from build123d import *

# Parameters (mm, degrees)
SKETCH1_W            = 8.5
SKETCH1_H            = 8.5
BOSS_EXTRUDE1_DEPTH  = 5
SKETCH2_W            = 8.5
SKETCH2_H            = 8.5
BOSS_EXTRUDE2_DEPTH  = 2
SKETCH3_R            = 1.5
CUT_EXTRUDE1_DEPTH   = 2
SKETCH4_W            = 82
SKETCH4_H            = 8.5
BOSS_EXTRUDE3_DEPTH  = 3
SKETCH5_W            = 7
SKETCH5_H            = 8.5
BOSS_EXTRUDE4_DEPTH  = 8.5
CUT_EXTRUDE2_DEPTH   = 5
SKETCH7_R            = 1.5
CUT_EXTRUDE3_DEPTH   = 5
CUT_EXTRUDE4_DEPTH   = 10
SKETCH9_W            = 8.5
SKETCH9_H            = 8.5
SKETCH9_R            = 1.5
BOSS_EXTRUDE5_DEPTH  = 2
CUT_EXTRUDE5_DEPTH   = 2
SKETCH11_W           = 8.5
SKETCH11_H           = 8.5
SKETCH11_R           = 1.5
BOSS_EXTRUDE6_DEPTH  = 2
BOSS_EXTRUDE7_DEPTH  = 5
BOSS_EXTRUDE8_DEPTH  = 5
SKETCH14_W           = 8.5
SKETCH14_H           = 11.5
CUT_EXTRUDE6_DEPTH   = 4
SKETCH15_W           = 8.5
SKETCH15_H           = 11.5
CUT_EXTRUDE7_DEPTH   = 4
SKETCH16_R           = 1.5
CUT_EXTRUDE8_DEPTH   = 4
SKETCH17_R           = 1.5
CUT_EXTRUDE9_DEPTH   = 4
SKETCH19_W           = 8.5
SKETCH19_H           = 8.5
BOSS_EXTRUDE9_DEPTH  = 3
SKETCH20_W           = 8.5
SKETCH20_H           = 8.5
BOSS_EXTRUDE10_DEPTH = 3


with BuildPart() as part:
    # Sketch1 → Boss-Extrude1 (new body)
    with BuildSketch(Plane(origin=(0, 0, 0), x_dir=(0, 0, -1), z_dir=(1, 0, 0))):
        Rectangle(SKETCH1_W, SKETCH1_H)
        Polygon((1.58771324, 2.75), (-1.58771324, 2.75), (-3.175426481, 0), (-1.58771324, -2.75), (1.58771324, -2.75), (3.175426481, 0), align=None, mode=Mode.SUBTRACT)
    extrude(amount=BOSS_EXTRUDE1_DEPTH)

    # Sketch2 → Boss-Extrude2 (add)
    with BuildSketch(Plane.ZY):
        Rectangle(SKETCH2_W, SKETCH2_H)
    extrude(amount=BOSS_EXTRUDE2_DEPTH)

    # Sketch3 → Cut-Extrude1 (cut)
    with BuildSketch(Plane(origin=(0, 0, 0), x_dir=(0, 0, -1), z_dir=(1, 0, 0))):
        Circle(SKETCH3_R)
    extrude(amount=-CUT_EXTRUDE1_DEPTH, mode=Mode.SUBTRACT)

    # Sketch4 → Boss-Extrude3 (add)
    with BuildSketch(Plane.XZ.offset(4.25)):
        with Locations((39, 0)):
            Rectangle(SKETCH4_W, SKETCH4_H)
    extrude(amount=BOSS_EXTRUDE3_DEPTH)

    # Sketch5 → Boss-Extrude4 (add)
    with BuildSketch(Plane(origin=(0, -4.25, 0), x_dir=(1, 0, 0), z_dir=(0, 1, 0))):
        with Locations((76.5, 0)):
            Rectangle(SKETCH5_W, SKETCH5_H)
    extrude(amount=BOSS_EXTRUDE4_DEPTH)

    # Sketch6 → Cut-Extrude2 (cut)
    with BuildSketch(Plane.ZY.offset(-73)):
        Polygon((3.175426481, 0), (1.58771324, 2.75), (-1.58771324, 2.75), (-3.175426481, 0), (-1.58771324, -2.75), (1.58771324, -2.75), align=None)
    extrude(amount=-CUT_EXTRUDE2_DEPTH, mode=Mode.SUBTRACT)

    # Sketch7 → Cut-Extrude3 (cut)
    with BuildSketch(Plane.ZY.offset(-78)):
        Circle(SKETCH7_R)
    extrude(amount=-CUT_EXTRUDE3_DEPTH, mode=Mode.SUBTRACT)

    # Sketch8 → Cut-Extrude4 (cut)
    with BuildSketch(Plane.ZY.offset(2)):
        Polygon((-1.58771324, 2.75), (1.58771324, 2.75), (3.175426481, 0), (1.58771324, -2.75), (-1.58771324, -2.75), (-3.175426481, 0), align=None)
    extrude(amount=-CUT_EXTRUDE4_DEPTH, mode=Mode.SUBTRACT)

    # Sketch9 → Boss-Extrude5 (add)
    with BuildSketch(Plane(origin=(5, 0, 0), x_dir=(0, 0, -1), z_dir=(1, 0, 0))):
        Rectangle(SKETCH9_W, SKETCH9_H)
        Circle(SKETCH9_R, mode=Mode.SUBTRACT)
    extrude(amount=-BOSS_EXTRUDE5_DEPTH)

    # Sketch10 → Cut-Extrude5 (cut)
    with BuildSketch(Plane(origin=(80, 0, 0), x_dir=(0, 0, -1), z_dir=(1, 0, 0))):
        Polygon((-3.175426481, 0), (-1.58771324, 2.75), (1.58771324, 2.75), (3.175426481, 0), (1.58771324, -2.75), (-1.58771324, -2.75), align=None)
    extrude(amount=-CUT_EXTRUDE5_DEPTH, mode=Mode.SUBTRACT)

    # Sketch11 → Boss-Extrude6 (add)
    with BuildSketch(Plane.ZY.offset(-73)):
        Rectangle(SKETCH11_W, SKETCH11_H)
        Circle(SKETCH11_R, mode=Mode.SUBTRACT)
    extrude(amount=-BOSS_EXTRUDE6_DEPTH)

    # Sketch12 → Boss-Extrude7 (add)
    with BuildSketch(Plane.ZY.offset(-3)):
        Polygon((-3.175426481, 0), (-1.58771324, 2.75), (1.58771324, 2.75), (3.175426481, 0), (1.58771324, -2.75), (-1.58771324, -2.75), align=None)
    extrude(amount=BOSS_EXTRUDE7_DEPTH)

    # Sketch13 → Boss-Extrude8 (add)
    with BuildSketch(Plane(origin=(75, 0, 0), x_dir=(0, 0, -1), z_dir=(1, 0, 0))):
        Polygon((-1.58771324, 2.75), (-3.175426481, 0), (-1.58771324, -2.75), (1.58771324, -2.75), (3.175426481, 0), (1.58771324, 2.75), align=None)
    extrude(amount=BOSS_EXTRUDE8_DEPTH)

    # Sketch14 → Cut-Extrude6 (cut)
    with BuildSketch(Plane.ZY.offset(2)):
        with Locations((0, -1.5)):
            Rectangle(SKETCH14_W, SKETCH14_H)
    extrude(amount=-CUT_EXTRUDE6_DEPTH, mode=Mode.SUBTRACT)

    # Sketch15 → Cut-Extrude7 (cut)
    with BuildSketch(Plane(origin=(80, 0, 0), x_dir=(0, 0, -1), z_dir=(1, 0, 0))):
        with Locations((0, -1.5)):
            Rectangle(SKETCH15_W, SKETCH15_H)
    extrude(amount=-CUT_EXTRUDE7_DEPTH, mode=Mode.SUBTRACT)

    # Sketch16 → Cut-Extrude8 (cut)
    with BuildSketch(Plane(origin=(5, 0, 0), x_dir=(0, 0, -1), z_dir=(1, 0, 0))):
        Circle(SKETCH16_R)
    extrude(amount=-CUT_EXTRUDE8_DEPTH, mode=Mode.SUBTRACT)

    # Sketch17 → Cut-Extrude9 (cut)
    with BuildSketch(Plane.ZY.offset(-75)):
        Circle(SKETCH17_R)
    extrude(amount=-CUT_EXTRUDE9_DEPTH, mode=Mode.SUBTRACT)

    # Sketch19 → Boss-Extrude9 (add)
    with BuildSketch(Plane(origin=(5, 0, 0), x_dir=(0, 0, -1), z_dir=(1, 0, 0))):
        Rectangle(SKETCH19_W, SKETCH19_H)
    extrude(amount=-BOSS_EXTRUDE9_DEPTH)

    # Sketch20 → Boss-Extrude10 (add)
    with BuildSketch(Plane.ZY.offset(-73)):
        Rectangle(SKETCH20_W, SKETCH20_H)
    extrude(amount=-BOSS_EXTRUDE10_DEPTH)


solid = part.part
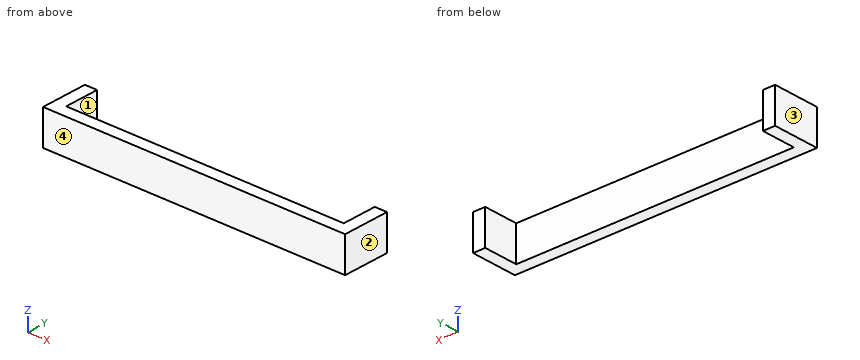
Design review of the part built by this model. Coordinates are the model's own, in mm. Face numbers are marked on the shaded views. Round coordinates to 2 decimals unless told otherwise and drop trailing zeros. Write each loop counter-clockwise with the first axis right and the second up, starting at its lowest first coordinate (ties: lowest second). Pieces come first, ordered by that corner, then holes.
Item 1: Draft analysis for pull direction X (two halves, no side actions). For the marked faces 1, 2, 3 and 4, state which applies: released by +X, released by -X, zero draft, split by the parting line, or undercut.
Item 2: Consider section B-B on z = -0.25. Give the boundary of the cut face in (x, y).
Item 3: Consider section A-A on y = 3.25. Give the boundary of the cut face in (x, z).
Item 4: For pin 1 Ø2.5 at (x, z) = (23.5, 1) entering from +Y, flat-tipped, find the tip position at first contact; note if it passes through.
Item 5: Consider section C-C on x = 42. Give the boundary of the cut face in (y, z).
Item 6: Wall thickness on L1, parallel to X at y = 3, z = 1.75; L2, parallel to Y at x = 21.5, z = 2.5: over which ranges is each line inside the solid? List them lowest first.
Check values:
1. face 1: undercut
1. face 2: released by +X
1. face 3: released by -X
1. face 4: zero draft
2. outline: (2, -7.25) - (76, -7.25) - (76, 4.25) - (73, 4.25) - (73, -4.25) - (5, -4.25) - (5, 4.25) - (2, 4.25) - close
3. outline: (2, -4.25) - (5, -4.25) - (5, 4.25) - (2, 4.25) - close; (73, -4.25) - (76, -4.25) - (76, 4.25) - (73, 4.25) - close
4. pin 1: stops at y = -4.25
5. outline: (-7.25, -4.25) - (-4.25, -4.25) - (-4.25, 4.25) - (-7.25, 4.25) - close
6. L1: x = 2 to 5, 73 to 76
6. L2: y = -7.25 to -4.25
